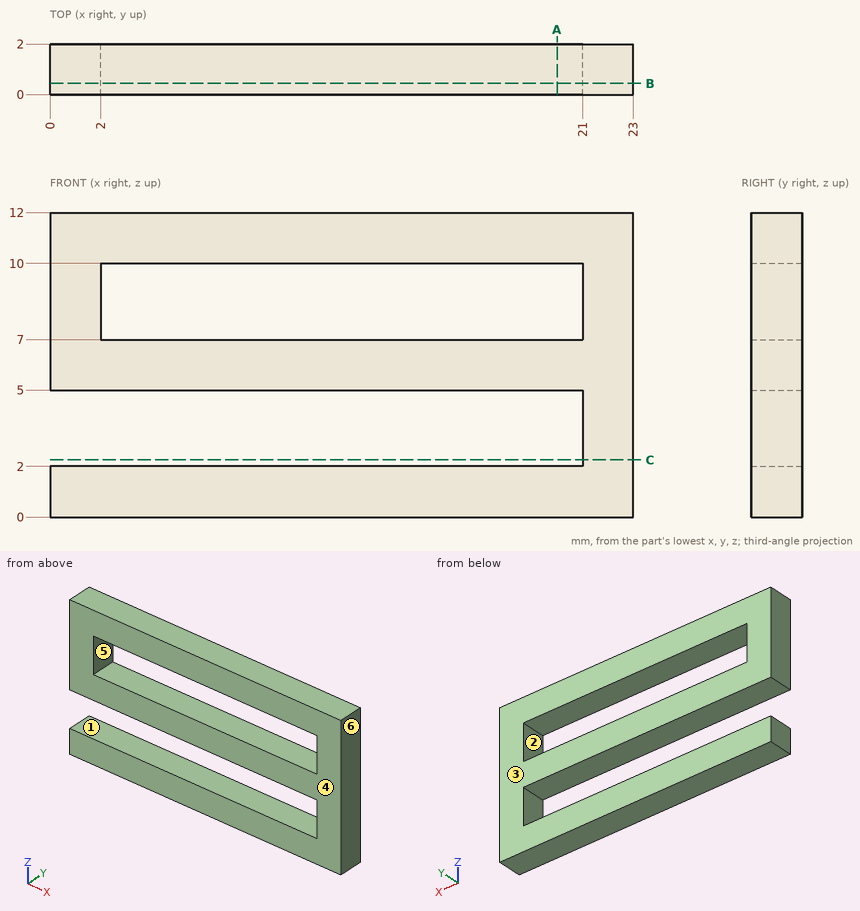
Geometry: see drawing. Coordinates: mm, zero at the bounding-box minimum. A direction names the side the tool comes from. Coordinates: 2 decimals unless noted, no trailing zeros. Loops run counter-clockwise (first coordinate to the right, second up) from the corner with the lowest first, then second, coordinate; pieces in that order, holes last.
Q1. Cut plane B-B (y = 0.45). Output: boundary loops of the cut face in (x, z), then the cut area to 3 significant figures.
Q2. Material intervals for line 1 (Z direction, x = 10.75, y = 0.7); line 2 (X direction, y = 0.35, z = 8.5); line 3 (Z direction, x = 1, y = 0.5), sorted ascending.
Q3. Set-up query: the marked faces 1, 2 and 3. Return all of +Z, -Z, +X, -X, +Y, -Y with unobstructed straight access to the full face (end or side cutting, diameter ignored); none if empty.
Q4. Cut plane A-A (x = 20). Output: boundary loops of the cut face in (y, z), then the cut area to 3 significant figures.
Q5. Cut plane C-C (z = 2.25). Output: boundary loops of the cut face in (x, y), then the cut area to 3 significant figures.
Q6. Draft query along X for the marked faces 4, 5 and 6. Return one class per face: +X half, -X half, draft (parallel to the pull), parting line (faces both ways), or undercut.
Working result:
1. outline: (0, 0) - (23, 0) - (23, 12) - (0, 12) - (0, 5) - (21, 5) - (21, 2) - (0, 2) - close; hole (2, 7) - (21, 7) - (21, 10) - (2, 10) - close
1. area: 156 mm2
2. line 1: z = 0 to 2, 5 to 7, 10 to 12
2. line 2: x = 0 to 2, 21 to 23
2. line 3: z = 0 to 2, 5 to 12
3. face 1: -X, +Y, -Y
3. face 2: +Y, -Y
3. face 3: +Z, -Z, +X, -X, +Y
4. outline: (0, 0) - (2, 0) - (2, 2) - (0, 2) - close; (0, 5) - (2, 5) - (2, 7) - (0, 7) - close; (0, 10) - (2, 10) - (2, 12) - (0, 12) - close
4. area: 12.0 mm2
5. outline: (21, 0) - (23, 0) - (23, 2) - (21, 2) - close
5. area: 4.00 mm2
6. face 4: draft
6. face 5: undercut
6. face 6: +X half
